```python
from build123d import *

# Parameters (mm, degrees)
SKETCH1_R           = 5
BOSS_EXTRUDE1_DEPTH = 30
SKETCH6_R           = 5
BOSS_EXTRUDE3_DEPTH = 5


with BuildPart() as part:
    # Sketch1 → Boss-Extrude1 (new body)
    with BuildSketch(Plane.XY):
        Circle(SKETCH1_R)
    extrude(amount=BOSS_EXTRUDE1_DEPTH)

    # Sketch6 → Boss-Extrude3 (add)
    # profile 1 of 2: a face of its own
    with BuildSketch(Plane.XY.offset(30)):
        Polygon((5, 8.660254038), (-5, 8.660254038), (-10, 0), (-5, -8.660254038), (5, -8.660254038), (10, 0), align=None)
        Circle(SKETCH6_R, mode=Mode.SUBTRACT)
    # profile 2 of 2: a face of its own
    with BuildSketch(Plane.XY.offset(30)):
        Circle(SKETCH6_R)
    extrude(amount=BOSS_EXTRUDE3_DEPTH)


solid = part.part
```
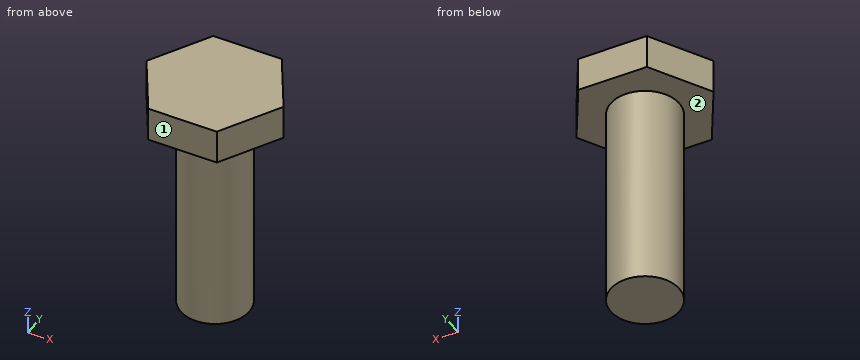
The model under review builds one solid part; all positions refer to its coordinate system, in mm. Face numbers are marked on the shaded views. A direction names the side the tool comes from. Round coordinates to 2 decimals unless told otherwise and drop trailing zeros. Order: outer loops, then holes, each group sorted by start corner. A loop starts at its lowest first (then second) coordinate and runs counter-clockwise, first axis right, second up. Notation, with made-up numbers: (-34, -26) -> (-11, -26) arc R8 ccw to (-11, -21) -> close; hole circle Ø9 at (75, 15). An arc over 180 degrees is marked (long way). One line per item, written item: value. Start each with the question number.
Q1. Take a section at C-C (z = 21.5). Write out the cut boundary in (x, y), and give its area (3 significant figures).
Q2. Machinability: for the marked faces 1 and 2, which of the approach directions +Z, -Z, +X, -X, +Y, -Y give a long, thin tool a straight path to every point of the face, cutting with its end or side? Answer none if there is none.
Q3. Take a section at A-A (x = 0). Write out the cut boundary in (y, z), and give its area (3 significant figures).
Q4. Take a section at D-D (x = -7.75). Write out the cut boundary in (y, z).
Q5. Wall thickness on line 1 (Z direction, x = 5.5, y = 2.25); line 2 (X direction, y = 3.75, z = 22.5); line 3 (X direction, y = 1.25, z = 10.5): over which ranges is each line inside the solid? List them lowest first.
Q6. Clearance check with flat-ended pins moving along their axes: pin 1 Ø5 at (x, z) = (-4.5, 8.5) entering from -Y; pin 2 Ø10 at (x, z) = (1, 5) entering from +Y; pin 3 Ø5 at (x, y) = (-1, -3.5) entering from -Z; pin 4 Ø3 at (x, y) = (-5, 7) entering from -Z. State where each tip first meets the part, or that it passes through.
Q7. Take a section at B-B (y = -4.25). Write out the cut boundary in (x, z), and give its area (3 significant figures).
Reported:
1. outline: circle Ø10 at (0, 0)
1. area: 78.5 mm2
2. face 1: +Z, -Z, +X, -X, -Y
2. face 2: -Z
3. outline: (-8.66, 30) -> (-5, 30) -> (-5, 0) -> (5, 0) -> (5, 30) -> (8.66, 30) -> (8.66, 35) -> (-8.66, 35) -> close
3. area: 387 mm2
4. outline: (-3.9, 30) -> (3.9, 30) -> (3.9, 35) -> (-3.9, 35) -> close
5. line 1: z = 30 to 35
5. line 2: x = -3.31 to 3.31
5. line 3: x = -4.84 to 4.84
6. pin 1: stops at y = -4.58
6. pin 2: stops at y = 5
6. pin 3: stops at z = 0
6. pin 4: stops at z = 30
7. outline: (-7.55, 30) -> (-2.63, 30) -> (-2.63, 0) -> (2.63, 0) -> (2.63, 30) -> (7.55, 30) -> (7.55, 35) -> (-7.55, 35) -> close
7. area: 233 mm2
